from build123d import *

# Parameters (mm, degrees)
SKETCH_1_W          = 80
SKETCH_1_H          = 97
SKETCH_1_R          = 1.5
EXTRUDE_1_DEPTH     = 3
SKETCH_3_W          = 32
SKETCH_3_H          = 62.377964324
EXTRUDE_2_DEPTH     = 3
EXTRUDE_3_DEPTH     = 3
SKETCH_5_R          = 1.5
CUT_EXTRUDE_2_DEPTH = 3
SKETCH_6_R          = 1.5
CUT_EXTRUDE_4_DEPTH = 3
FILLET_1_R          = 5
FILLET_2_R          = 5
CUT_EXTRUDE_5_DEPTH = 10
SKETCH_9_W          = 35.553305852
SKETCH_9_H          = 40.684386559
EXTRUDE_4_DEPTH     = 3
CUT_EXTRUDE_6_REACH = 159.896
SKETCH_10_R         = 1.5
CUT_EXTRUDE_7_REACH = 159.896
SKETCH_11_R         = 1.5


with BuildPart() as part:
    # 草图1 → 凸台-拉伸1 (new body)
    with BuildSketch(Plane.XY):
        with Locations((33.620020091, -43.208150262)):
            Rectangle(SKETCH_1_W, SKETCH_1_H)
        Circle(SKETCH_1_R, mode=Mode.SUBTRACT)
        with Locations((66.99974208, 0.185906473)):
            Circle(SKETCH_1_R, mode=Mode.SUBTRACT)
        with Locations((5.231118743, -83.287075899)):
            Circle(SKETCH_1_R, mode=Mode.SUBTRACT)
        with Locations((62.230899318, -83.128916661)):
            Circle(SKETCH_1_R, mode=Mode.SUBTRACT)
    extrude(amount=EXTRUDE_1_DEPTH)

    # 草图3 → 凸台-拉伸2 (add)
    with BuildSketch(Plane.XY.offset(3)):
        with Locations((-22.379979909, -57.897132424)):
            Rectangle(SKETCH_3_W, SKETCH_3_H)
        with Locations((89.620020091, -57.897132424)):
            Rectangle(SKETCH_3_W, SKETCH_3_H)
    extrude(amount=-EXTRUDE_2_DEPTH)

    # 草图4 → 凸台-拉伸3 (add)
    with BuildSketch(Plane.XY.offset(3)):
        Polygon((-38.379979909, -89.086114586), (-38.379979909, -106.898150262), (-4.25, -106.898150262), (-0.590540516, -106.898150262), (-0.590540516, -117.135828938), (20.473808019, -117.135828938), (46.526191981, -117.135828938), (67.71, -117.391270189), (67.71, -106.991270189), (71.25, -106.991270189), (105.5, -106.991270189), (105.5, -89.086114586), (72.50067844, -84.475650121), (55.009126254, -90.348726038), (11.990873746, -90.348726038), (-5.50067844, -84.475650121), align=None)
    extrude(amount=-EXTRUDE_3_DEPTH)

    # 草图5 → 切除-拉伸2 (cut)
    with BuildSketch(Plane.XY.offset(3)):
        with Locations((-27.629979909, -38.388150262)):
            Circle(SKETCH_5_R)
        with Locations((-7.879979909, -38.388150262)):
            Circle(SKETCH_5_R)
        with Locations((-27.629979909, -95.218150262)):
            Circle(SKETCH_5_R)
        with Locations((-7.879979909, -95.218150262)):
            Circle(SKETCH_5_R)
        with Locations(Location((75.120020091, -95.218150262, 0), (0, 0, 180))):
            Circle(SKETCH_5_R)
        with Locations(Location((94.870020091, -95.218150262, 0), (0, 0, 180))):
            Circle(SKETCH_5_R)
        with Locations(Location((75.120020091, -38.388150262, 0), (0, 0, 180))):
            Circle(SKETCH_5_R)
        with Locations(Location((94.870020091, -38.388150262, 0), (0, 0, 180))):
            Circle(SKETCH_5_R)
    extrude(amount=-CUT_EXTRUDE_2_DEPTH, mode=Mode.SUBTRACT)

    # 草图6 → 切除-拉伸4 (cut)
    with BuildSketch(Plane.XY.offset(3)):
        with Locations((12.030020091, -20.143150262)):
            Circle(SKETCH_6_R)
        with Locations((55.210020091, -20.143150262)):
            Circle(SKETCH_6_R)
        with Locations((12.030020091, -76.273150262)):
            Circle(SKETCH_6_R)
        with Locations((55.210020091, -76.273150262)):
            Circle(SKETCH_6_R)
    extrude(amount=-CUT_EXTRUDE_4_DEPTH, mode=Mode.SUBTRACT)

    # 圆角1
    fillet_1_edges = [part.edges().sort_by_distance(p)[0] for p in [
        (-6.379979909, 5.291849738, 1.5),
        (73.620020091, 5.291849738, 1.5),
        (-6.379979909, -26.708150262, 1.5),
        (-38.379979909, -26.708150262, 1.5),
        (105.620020091, -26.708150262, 1.5),
        (73.620020091, -26.708150262, 1.5),
        (105.5, -106.991270189, 1.5),
        (67.71, -106.991270189, 1.5),
        (-0.590540516, -117.135828938, 1.5),
        (-0.590540516, -106.898150262, 1.5),
        (-38.379979909, -106.898150262, 1.5),
    ]]
    fillet(fillet_1_edges, radius=FILLET_1_R)

    # 圆角2
    fillet_2_edges = [part.edges().sort_by_distance(p)[0] for p in [
        (67.71, -117.391270189, 1.5),
    ]]
    fillet(fillet_2_edges, radius=FILLET_2_R)

    # 草图8 → 切除-拉伸5 (cut)
    with BuildSketch(Plane.XY.offset(3)):
        with BuildLine():
            Line((-25.629979909, -42.884254011), (-9.879979909, -42.884254011))
            ThreePointArc((-9.879979909, -42.884254011), (-8.465766346, -43.470040449), (-7.879979909, -44.884254011))
            Line((-7.879979909, -44.884254011), (-7.879979909, -88.722046513))
            ThreePointArc((-7.879979909, -88.722046513), (-8.465766346, -90.136260075), (-9.879979909, -90.722046513))
            Line((-9.879979909, -90.722046513), (-25.629979909, -90.722046513))
            ThreePointArc((-25.629979909, -90.722046513), (-27.044193471, -90.136260075), (-27.629979909, -88.722046513))
            Line((-27.629979909, -88.722046513), (-27.629979909, -44.884254011))
            ThreePointArc((-27.629979909, -44.884254011), (-27.044193471, -43.470040449), (-25.629979909, -42.884254011))
        make_face()
        with BuildLine():
            Line((20.981769159, -2.213743129), (47.098456354, -2.213743129))
            ThreePointArc((47.098456354, -2.213743129), (48.512669916, -2.799529566), (49.098456354, -4.213743129))
            Line((49.098456354, -4.213743129), (49.098456354, -35.822296813))
            ThreePointArc((49.098456354, -35.822296813), (49.684242792, -37.236510375), (51.098456354, -37.822296813))
            Line((51.098456354, -37.822296813), (63.396898836, -37.822296813))
            ThreePointArc((63.396898836, -37.822296813), (64.811112398, -38.40808325), (65.396898836, -39.822296813))
            Line((65.396898836, -39.822296813), (65.396898836, -68.419181777))
            ThreePointArc((65.396898836, -68.419181777), (64.811112398, -69.833395339), (63.396898836, -70.419181777))
            Line((63.396898836, -70.419181777), (51.098456354, -70.419181777))
            ThreePointArc((51.098456354, -70.419181777), (49.684242792, -71.004968215), (49.098456354, -72.419181777))
            Line((49.098456354, -72.419181777), (49.098456354, -104.027735461))
            ThreePointArc((49.098456354, -104.027735461), (48.512669916, -105.441949023), (47.098456354, -106.027735461))
            Line((47.098456354, -106.027735461), (20.981769159, -106.027735461))
            ThreePointArc((20.981769159, -106.027735461), (19.567555596, -105.441949023), (18.981769159, -104.027735461))
            Line((18.981769159, -104.027735461), (18.981769159, -72.419181777))
            ThreePointArc((18.981769159, -72.419181777), (18.395982721, -71.004968215), (16.981769159, -70.419181777))
            Line((16.981769159, -70.419181777), (4.683326676, -70.419181777))
            ThreePointArc((4.683326676, -70.419181777), (3.269113114, -69.833395339), (2.683326676, -68.419181777))
            Line((2.683326676, -68.419181777), (2.683326676, -39.822296813))
            ThreePointArc((2.683326676, -39.822296813), (3.269113114, -38.40808325), (4.683326676, -37.822296813))
            Line((4.683326676, -37.822296813), (16.981769159, -37.822296813))
            ThreePointArc((16.981769159, -37.822296813), (18.395982721, -37.236510375), (18.981769159, -35.822296813))
            Line((18.981769159, -35.822296813), (18.981769159, -4.213743129))
            ThreePointArc((18.981769159, -4.213743129), (19.567555596, -2.799529566), (20.981769159, -2.213743129))
        make_face()
        with BuildLine():
            Line((93.710205421, -90.722046513), (77.960205421, -90.722046513))
            ThreePointArc((77.960205421, -90.722046513), (76.545991859, -90.136260075), (75.960205421, -88.722046513))
            Line((75.960205421, -88.722046513), (75.960205421, -44.884254011))
            ThreePointArc((75.960205421, -44.884254011), (76.545991859, -43.470040449), (77.960205421, -42.884254011))
            Line((77.960205421, -42.884254011), (93.710205421, -42.884254011))
            ThreePointArc((93.710205421, -42.884254011), (95.124418984, -43.470040449), (95.710205421, -44.884254011))
            Line((95.710205421, -44.884254011), (95.710205421, -88.722046513))
            ThreePointArc((95.710205421, -88.722046513), (95.124418984, -90.136260075), (93.710205421, -90.722046513))
        make_face()
    extrude(amount=-CUT_EXTRUDE_5_DEPTH, mode=Mode.SUBTRACT)

    # 草图9 → 凸台-拉伸4 (add)
    with BuildSketch(Plane.XY.offset(3)):
        with Locations((35.048637375, -17.480103533)):
            Rectangle(SKETCH_9_W, SKETCH_9_H)
    extrude(amount=-EXTRUDE_4_DEPTH)

    # 草图10 → 切除-拉伸6 (cut, up to next)
    with BuildSketch(Plane.XY.offset(3), mode=Mode.PRIVATE) as cut_extrude_6_sk1:
        with Locations((6.370020091, -26.298500215)):
            Circle(SKETCH_10_R)
    cut_extrude_6_tool1 = extrude(cut_extrude_6_sk1.sketch, amount=-CUT_EXTRUDE_6_REACH, mode=Mode.PRIVATE) & part.part
    # 草图10 → 切除-拉伸6 (cut, up to next)
    with BuildSketch(Plane.XY.offset(3), mode=Mode.PRIVATE) as cut_extrude_6_sk2:
        with Locations((60.870020091, -26.298500215)):
            Circle(SKETCH_10_R)
    cut_extrude_6_tool2 = extrude(cut_extrude_6_sk2.sketch, amount=-CUT_EXTRUDE_6_REACH, mode=Mode.PRIVATE) & part.part
    # 草图10 → 切除-拉伸6 (cut, up to next)
    with BuildSketch(Plane.XY.offset(3), mode=Mode.PRIVATE) as cut_extrude_6_sk3:
        with Locations((6.370020091, -99.798500215)):
            Circle(SKETCH_10_R)
    cut_extrude_6_tool3 = extrude(cut_extrude_6_sk3.sketch, amount=-CUT_EXTRUDE_6_REACH, mode=Mode.PRIVATE) & part.part
    # 草图10 → 切除-拉伸6 (cut, up to next)
    with BuildSketch(Plane.XY.offset(3), mode=Mode.PRIVATE) as cut_extrude_6_sk4:
        with Locations((60.870020091, -99.798500215)):
            Circle(SKETCH_10_R)
    cut_extrude_6_tool4 = extrude(cut_extrude_6_sk4.sketch, amount=-CUT_EXTRUDE_6_REACH, mode=Mode.PRIVATE) & part.part
    add(cut_extrude_6_tool1.solids().sort_by_distance((6.37002, -26.2985, 3))[0], mode=Mode.SUBTRACT)
    add(cut_extrude_6_tool2.solids().sort_by_distance((60.87002, -26.2985, 3))[0], mode=Mode.SUBTRACT)
    add(cut_extrude_6_tool3.solids().sort_by_distance((6.37002, -99.7985, 3))[0], mode=Mode.SUBTRACT)
    add(cut_extrude_6_tool4.solids().sort_by_distance((60.87002, -99.7985, 3))[0], mode=Mode.SUBTRACT)

    # 草图11 → 切除-拉伸7 (cut, up to next)
    with BuildSketch(Plane.XY.offset(3), mode=Mode.PRIVATE) as cut_extrude_7_sk1:
        with Locations((26.195020091, -2.714801131)):
            Circle(SKETCH_11_R)
    cut_extrude_7_tool1 = extrude(cut_extrude_7_sk1.sketch, amount=-CUT_EXTRUDE_7_REACH, mode=Mode.PRIVATE) & part.part
    # 草图11 → 切除-拉伸7 (cut, up to next)
    with BuildSketch(Plane.XY.offset(3), mode=Mode.PRIVATE) as cut_extrude_7_sk2:
        with Locations((41.045020091, -2.714801131)):
            Circle(SKETCH_11_R)
    cut_extrude_7_tool2 = extrude(cut_extrude_7_sk2.sketch, amount=-CUT_EXTRUDE_7_REACH, mode=Mode.PRIVATE) & part.part
    # 草图11 → 切除-拉伸7 (cut, up to next)
    with BuildSketch(Plane.XY.offset(3), mode=Mode.PRIVATE) as cut_extrude_7_sk3:
        with Locations((26.195020091, -17.564801131)):
            Circle(SKETCH_11_R)
    cut_extrude_7_tool3 = extrude(cut_extrude_7_sk3.sketch, amount=-CUT_EXTRUDE_7_REACH, mode=Mode.PRIVATE) & part.part
    # 草图11 → 切除-拉伸7 (cut, up to next)
    with BuildSketch(Plane.XY.offset(3), mode=Mode.PRIVATE) as cut_extrude_7_sk4:
        with Locations((41.045020091, -17.564801131)):
            Circle(SKETCH_11_R)
    cut_extrude_7_tool4 = extrude(cut_extrude_7_sk4.sketch, amount=-CUT_EXTRUDE_7_REACH, mode=Mode.PRIVATE) & part.part
    add(cut_extrude_7_tool1.solids().sort_by_distance((26.19502, -2.714801, 3))[0], mode=Mode.SUBTRACT)
    add(cut_extrude_7_tool2.solids().sort_by_distance((41.04502, -2.714801, 3))[0], mode=Mode.SUBTRACT)
    add(cut_extrude_7_tool3.solids().sort_by_distance((26.19502, -17.564801, 3))[0], mode=Mode.SUBTRACT)
    add(cut_extrude_7_tool4.solids().sort_by_distance((41.04502, -17.564801, 3))[0], mode=Mode.SUBTRACT)


solid = part.part
The model under review builds one solid part; all positions refer to its coordinate system, in mm. A direction names the side the tool comes from. Give positions to 0.01 mm unless a question says otherwise; leave off trailing zeros. Order: outer loops, then holes, each group sorted by start corner. A loop starts at its lowest first (then second) coordinate and runs counter-clockwise, first axis right, second up. Notation, with made-up numbers: (-10, -14) -> (-4, -14) arc R11 ccw to (-4, -8) -> close; hole circle Ø2 at (-10.5, -38.75). An arc over 180 degrees is marked (long way). Write item = value, one per line. Start each with the question number.
(1) Draft analysis for pull direction Y (two halves, no side actions). For faces 4 (the cylindrical face through (93.44, -38.84, 1.52)), 5 (the flat face through (-6.38, -11, 1)), 6 (the cylindrical face through (69.21, -108.42, 1.48)), state which applies: +Y half, -Y half, draft (parallel to the pull), parting line (faces both ways), or undercut.
(2) Take a section at C-C (x = 90.5). Write out the cut boundary in (y, z).
(3) Take a section at A-A (y = -46.5). Write out the cut boundary in (x, z).
(4) For pin 1 Ø0.9 at (x, z) = (-16.5, 1) entering from +Y; pin 2 Ø1.8 at (x, y) = (-7.88, -95.22) entering from +Z, all flat-tipped, find the tip position at first contact; note any pin that passes through.
(5) For L1, parallel to X at y = -95, z = 1.35; L2, parallel to X at y = -99.5, z = 0.6; L3, parallel to X at y = -68.5, z = 1.5, list the stretches that pass through material, from the lowest coordinate up. Write a range as from..to.
(6) Take a section at D-D (z = 1.5). State how many separate pieces and enclosed holes the cut face has, plus the area to 3 significant figures.
(7) Tool access review of faces 1 (the flat face through (105.62, -61, 2)), 2 (the flat face through (89, -26.708, 2)), 3 (the flat face through (-18, -90.722, 2)): name each direction out of +Z, -Z, +X, -X, +Y, -Y from which nothing blocks a thin tool from reaching the whole face with its end or side.
(8) Take a section at B-B (x = -24). Write out the cut boundary in (y, z).
Returned:
q1.face_4 = undercut
q1.face_5 = draft
q1.face_6 = -Y half
q2.outline = (-106.99, 0) -> (-90.72, 0) -> (-90.72, 3) -> (-106.99, 3) -> close; (-42.88, 0) -> (-26.71, 0) -> (-26.71, 3) -> (-42.88, 3) -> close
q3.outline = (-38.38, 0) -> (-27.63, 0) -> (-27.63, 3) -> (-38.38, 3) -> close; (-7.88, 0) -> (2.68, 0) -> (2.68, 3) -> (-7.88, 3) -> close; (65.4, 0) -> (75.96, 0) -> (75.96, 3) -> (65.4, 3) -> close; (95.71, 0) -> (105.62, 0) -> (105.62, 3) -> (95.71, 3) -> close
q4.pin_1 = -26.71
q4.pin_2 = through
q5.L1 = -38.38..-29.11, -26.15..-9.36, -6.4..18.98, 49.1..73.64, 76.6..93.39, 96.35..105.5
q5.L2 = -38.38..4.9, 7.84..18.98, 49.1..59.4, 62.34..105.5
q5.L3 = -38.38..-27.63, -7.88..2.68, 65.4..75.96, 95.71..105.62
q6.separate_pieces = 1
q6.enclosed_holes = 27
q6.area = 9,620 mm²
q7.face_1 = +Z, -Z, +X, +Y, -Y
q7.face_2 = +Z, -Z, +X, +Y
q7.face_3 = +Z, -Z
q8.outline = (-106.9, 0) -> (-90.72, 0) -> (-90.72, 3) -> (-106.9, 3) -> close; (-42.88, 0) -> (-26.71, 0) -> (-26.71, 3) -> (-42.88, 3) -> close
